Input: part model. Units: mm. Frame: model coordinates. Face numbers are marked on the shaded views. A direction names the side the tool comes from. Coordinates: 2 decimals unless noted, no trailing zeros. Order: outer loops, then holes, each group sorted by start corner. A loop starts at its lowest first (then second) coordinate and runs counter-clockwise, first axis right, second up. Notation, with made-up numbers: (73.25, 52) -> (100.25, 52) arc R8 cw to (100.25, 64) -> close; hole circle Ø4 at (80, 45). An arc over 180 degrees is marked (long way). Write each question's results on one line, items separated by ' | '.
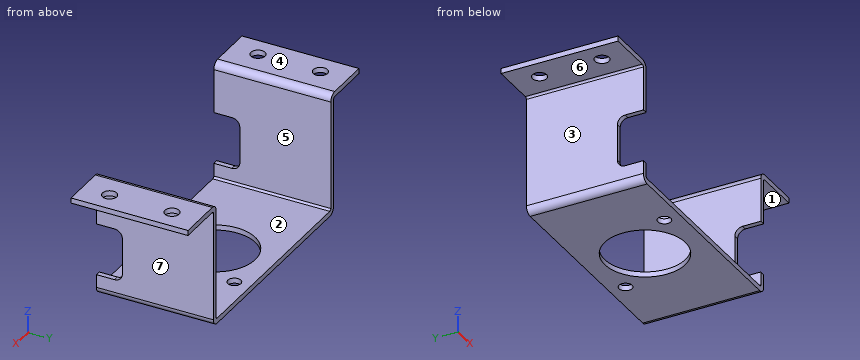
```python
from build123d import *

# Parameters (mm, degrees)
SKETCH2_W               = 80
SKETCH2_H               = 45
BASE_FLANGE1_DEPTH      = 2
EDGE_FLANGE1_DEPTH      = 45
EDGE_FLANGE2_DEPTH      = 45
SKETCH13_R              = 15.5
CUT_EXTRUDE1_DEPTH      = 65.440224857
SKETCH14_R              = 2.5
CUT_EXTRUDE2_DEPTH      = 65.440224857
EDGE_FLANGE3_DEPTH      = 45
EDGE_FLANGE3_BEND_DEPTH = 45
SKETCH21_R              = 2.75
CUT_EXTRUDE3_DEPTH      = 81.259717612
CUT_EXTRUDE4_DEPTH      = 116.211997682


# Sheet-metal steps are written as plain solids
with BuildPart() as part:
    # Sketch2 → Base-Flange1 (new body)
    with BuildSketch(Plane.XY):
        Rectangle(SKETCH2_W, SKETCH2_H)
    extrude(amount=-BASE_FLANGE1_DEPTH)

    # Edge-Flange1 section (across the edge) → Edge-Flange1 (add)
    with BuildSketch(Plane(origin=(40.7366, -22.5, 0), x_dir=(-1, 0, 0), z_dir=(0, 1, 0))):
        with BuildLine():
            Line((-2, 0.7366), (-2, 42.66))
            Line((-2, 42.66), (0, 42.66))
            Line((0, 42.66), (0, 0.7366))
            ThreePointArc((0, 0.7366), (0.215745145, 0.215745145), (0.7366, 0))
            Line((0.7366, 0), (0.7366, -2))
            ThreePointArc((0.7366, -2), (-1.198468417, -1.198468417), (-2, 0.7366))
        make_face()
    extrude(amount=EDGE_FLANGE1_DEPTH)

    # Edge-Flange2 section (across the edge) → Edge-Flange2 (add)
    with BuildSketch(Plane(origin=(-40.7366, 22.5, 0), x_dir=(1, 0, 0), z_dir=(0, -1, 0))):
        with BuildLine():
            Line((-2, 0.7366), (-2, 42.66))
            Line((-2, 42.66), (0, 42.66))
            Line((0, 42.66), (0, 0.7366))
            ThreePointArc((0, 0.7366), (0.215745145, 0.215745145), (0.7366, 0))
            Line((0.7366, 0), (0.7366, -2))
            ThreePointArc((0.7366, -2), (-1.198468417, -1.198468417), (-2, 0.7366))
        make_face()
    extrude(amount=EDGE_FLANGE2_DEPTH)

    # Sketch13 → Cut-Extrude1 (cut, through all)
    with BuildSketch(Plane.XY):
        Circle(SKETCH13_R)
    extrude(amount=-CUT_EXTRUDE1_DEPTH, mode=Mode.SUBTRACT)

    # Sketch14 → Cut-Extrude2 (cut, through all)
    with BuildSketch(Plane.XY):
        with Locations((-16.263455967, -16.263455967)):
            Circle(SKETCH14_R)
        with Locations((16.263455967, 16.263455967)):
            Circle(SKETCH14_R)
    extrude(amount=-CUT_EXTRUDE2_DEPTH, mode=Mode.SUBTRACT)

    # Edge-Flange3 section (across the edge) → Edge-Flange3 (add)
    with BuildSketch(Plane(origin=(42.7366, 22.5, 43.3966), x_dir=(0, 0, -1), z_dir=(0, -1, 0))):
        with BuildLine():
            Line((-2, 0.7366), (-2, 18))
            Line((-2, 18), (0, 18))
            Line((0, 18), (0, 0.7366))
            ThreePointArc((0, 0.7366), (0.215745145, 0.215745145), (0.7366, 0))
            Line((0.7366, 0), (0.7366, -2))
            ThreePointArc((0.7366, -2), (-1.198468417, -1.198468417), (-2, 0.7366))
        make_face()
    extrude(amount=EDGE_FLANGE3_DEPTH)

    # Edge-Flange3 section 2 (across the edge) → Edge-Flange3 bend (add)
    with BuildSketch(Plane(origin=(-42.7366, -22.5, 43.3966), x_dir=(0, 0, -1), z_dir=(0, 1, 0))):
        with BuildLine():
            Line((-2, 0.7366), (-2, 18))
            Line((-2, 18), (0, 18))
            Line((0, 18), (0, 0.7366))
            ThreePointArc((0, 0.7366), (0.215745145, 0.215745145), (0.7366, 0))
            Line((0.7366, 0), (0.7366, -2))
            ThreePointArc((0.7366, -2), (-1.198468417, -1.198468417), (-2, 0.7366))
        make_face()
    extrude(amount=EDGE_FLANGE3_BEND_DEPTH)

    # Sketch21 → Cut-Extrude3 (cut, through all)
    with BuildSketch(Plane.XY.offset(45.3966)):
        with Locations((52.7366, 12)):
            Circle(SKETCH21_R)
        with Locations((52.7366, -12)):
            Circle(SKETCH21_R)
        with Locations((-52.7366, 12)):
            Circle(SKETCH21_R)
        with Locations((-52.7366, -12)):
            Circle(SKETCH21_R)
    extrude(amount=-CUT_EXTRUDE3_DEPTH, mode=Mode.SUBTRACT)

    # Sketch22 → Cut-Extrude4 (cut, through all)
    with BuildSketch(Plane(origin=(42.7366, 0, 0), x_dir=(0, 0, -1), z_dir=(1, 0, 0))):
        with BuildLine():
            Line((-5.7366, -22.5), (-25.7366, -22.5))
            Line((-25.7366, -22.5), (-25.7366, -15.5))
            ThreePointArc((-25.7366, -15.5), (-24.857920344, -13.378679656), (-22.7366, -12.5))
            Line((-22.7366, -12.5), (-8.7366, -12.5))
            ThreePointArc((-8.7366, -12.5), (-6.615279656, -13.378679656), (-5.7366, -15.5))
            Line((-5.7366, -15.5), (-5.7366, -22.5))
        make_face()
    extrude(amount=-CUT_EXTRUDE4_DEPTH, mode=Mode.SUBTRACT)


solid = part.part
```
(1) Cut plane D-D, the plane y = 12. Count the separate pieces of the cut face and the enclosed holes in it, plus the area to 3 significant figures.
Return value:
separate pieces: 4 | enclosed holes: 0 | area: 357 mm2
(2) Cut plane A-A, the plane z = 3.5. Return loops of the section in (x, y), plus the area to 3 significant figures.
Return value:
outline: (-42.74, -22.5) -> (-40.74, -22.5) -> (-40.74, 22.5) -> (-42.74, 22.5) -> close; (40.74, -22.5) -> (42.74, -22.5) -> (42.74, 22.5) -> (40.74, 22.5) -> close | area: 180 mm2
(3) Cut plane C-C, the plane y = 0. Return loops of the section in (x, z).
Return value:
outline: (-60.74, 43.4) -> (-43.47, 43.4) arc R0.74 cw to (-42.74, 42.66) -> (-42.74, 0.74) arc R2.74 ccw to (-40, -2) -> (-15.5, -2) -> (-15.5, 0) -> (-40, 0) arc R0.74 cw to (-40.74, 0.74) -> (-40.74, 42.66) arc R2.74 ccw to (-43.47, 45.4) -> (-60.74, 45.4) -> close; (15.5, -2) -> (40, -2) arc R2.74 ccw to (42.74, 0.74) -> (42.74, 42.66) arc R0.74 cw to (43.47, 43.4) -> (60.74, 43.4) -> (60.74, 45.4) -> (43.47, 45.4) arc R2.74 ccw to (40.74, 42.66) -> (40.74, 0.74) arc R0.74 cw to (40, 0) -> (15.5, 0) -> close
(4) Line query: line 1 along X through (y, z) = (9, 40); line 2 along Y through (x, z) = (0, -1); line 3 along Z through (x, y) = (52, 1.5). Output: solid intervals per line, ascending. Write a range as from..to.
Return value:
line 1: -42.74..-40.74, 40.74..42.74 | line 2: -22.5..-15.5, 15.5..22.5 | line 3: 43.4..45.4
(5) Mould query, pull axis X, two halves, no side actions, for the marked faces 5, 6 and 7. Classes: +X half, -X half, draft (parallel to the pull), parting line (faces both ways), or undercut.
Return value:
face 5: undercut | face 6: draft | face 7: +X half
(6) Pin query (flat end, axial travel): P1, Ø2, axis at x = 42, y = -17.5, coming from the -Z side; P2, Ø1.6, axis at x = -42, y = -17.5, coming from the -Z side; P3, Ø8.5, axis at x = -56, y = 0.5, coming from the -Z side. Return the tip coordinate at first contact, or that it passes through.
Return value:
P1: z = -1.81 | P2: z = -1.72 | P3: z = 43.4
(7) Reachability of the marked faces 1, 2, 3 and 4 from +Z, -Z, +X, -X, +Y, -Y: full face, straight path, thin tool, end or side. Return the list, or none.
Return value:
face 1: -Z, +X, +Y, -Y | face 2: +Z, +Y, -Y | face 3: -Z, -X, +Y, -Y | face 4: +Z, +X, -X, +Y, -Y
(8) Cut plane B-B, the plane x = 0. Return loops of the section in (y, z).
Return value:
outline: (-22.5, -2) -> (-15.5, -2) -> (-15.5, 0) -> (-22.5, 0) -> close; (15.5, -2) -> (22.5, -2) -> (22.5, 0) -> (15.5, 0) -> close
